Could you check a few things on this model? Use its own coordinates, in mm. Face numbers are marked on the shaded views. A direction names the side the tool comes from. Give positions to 0.01 mm unless a question says otherwise; leave off trailing zeros. Loops run counter-clockwise (first coordinate to the right, second up) from the corner with the lowest first, then second, coordinate; pieces in that order, holes last. Notation, with made-up numbers: (36.25, 40.25) - (58.25, 40.25) arc R10 ccw to (58.25, 57.25) - close; hole circle Ø5 at (74, -26.75). An arc over 180 degrees is marked (long way). One line per item, written item: value. Start each with the question number.
Q1. If I drill on line 1 (Z direction, x = 11, y = -428.5); line 2 (X direction, y = -446, z = 324.5); line 3 (Z direction, x = 118.5, y = -600), over which ranges is the centre line in solid material (lowest first)? Write a range as from..to.
Q2. I want a section at A-A (z = 465.5). Please give me the cut outline in (x, y), then the cut area to 3 significant figures.
Q3. I want a section at C-C (y = -469). Please give me the cut outline in (x, z), then the cut area to 3 significant figures.
Q4. For the marked faces 1, 2 and 3, which set-ups out of +Z, -Z, +X, -X, +Y, -Y let a thin tool reach every point of the face, with its end or its side?
Q5. I want a section at D-D (z = 618). Please give me the cut outline in (x, y).
Q6. I want a section at B-B (x = 69). Please give me the cut outline in (y, z), then the cut area to 3 significant figures.
Q7. I'm going to push flat-ended pins straight in: P1, Ø12, axis at x = -387.5, z = 736.5, coming from the -Y side; P2, Ø5, axis at x = 190, y = -269, coming from the -Z side. Where does each tip first touch, or does it pass through?
Q8. If we mould it in two halves opening along X, with no side actions, what happens to the marked faces 4, 5, 6 and 7? For each: released by +X, released by -X, zero draft, split by the parting line, or undercut.
```python
from build123d import *

# Parameters (mm, degrees)
F1_DEPTH  = 500
F3_W      = 50
F3_H      = 50
F4_DEPTH  = 650
F5_W      = 50
F5_H      = 50
F6_DEPTH  = 200
F8_W      = 1200
F8_H      = 18
F9_DEPTH  = 150
F11_DEPTH = 1164


with BuildPart() as f1:
    # F0 (on Front) → F1 (new body)
    with BuildSketch(Plane.XZ):
        Polygon((0, 1115), (-600, 1115), (-600, 200), (0, 200), (0, 218), (-582, 218), (-582, 1097), (0, 1097), align=None)
    extrude(amount=F1_DEPTH)

    # F3 (on offset) → F4 (join)
    with BuildSketch(Plane.XZ):
        with Locations((-575, 175)):
            Rectangle(F3_W, F3_H)
    extrude(amount=F4_DEPTH)

    # F5 (on Top) → F6 (join)
    with BuildSketch(Plane.XY):
        with Locations((-575, -25)):
            Rectangle(F5_W, F5_H)
        with Locations((-575, -625)):
            Rectangle(F5_W, F5_H)
    extrude(amount=F6_DEPTH)

    # F7: F1 across plane


with BuildPart() as f1_1:
    add(f1.part)
    add(f1.part.mirror(Plane.YZ))

    # F8 (on face) → F9 (join)
    with BuildSketch(Plane.XZ.offset(500)):
        with Locations((0, 1106)):
            Rectangle(F8_W, F8_H)
    extrude(amount=F9_DEPTH)

    # F10 (on face) → F11 (join, through all)
    with BuildSketch(Plane.YZ.offset(-582)):
        Polygon((0, 897), (-500, 897), (-500, 879), (-18, 879), (-18, 568), (-500, 568), (-500, 550), (0, 550), align=None)
    extrude(amount=F11_DEPTH)


solid = f1_1.part
```
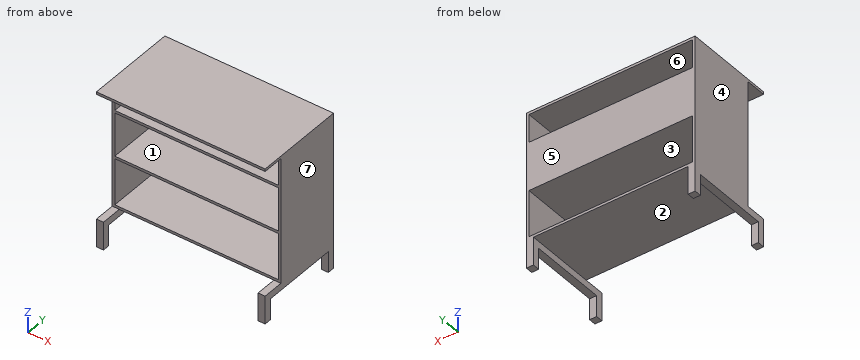
Worked answers:
1. line 1: z = 200..218, 550..568, 879..897, 1097..1115
1. line 2: x = -600..-582, 582..600
1. line 3: z = 1097..1115
2. outline: (-600, -500) - (-582, -500) - (-582, 0) - (-600, 0) - close; (582, -500) - (600, -500) - (600, 0) - (582, 0) - close
2. area: 18,000 mm²
3. outline: (-600, 150) - (-550, 150) - (-550, 200) - (550, 200) - (550, 150) - (600, 150) - (600, 1115) - (-600, 1115) - close; hole (-582, 218) - (582, 218) - (582, 550) - (-582, 550) - close; hole (-582, 568) - (582, 568) - (582, 879) - (-582, 879) - close; hole (-582, 897) - (582, 897) - (582, 1097) - (-582, 1097) - close
3. area: 122,000 mm²
4. face 1: -Y
4. face 2: -Z, +Y, -Y
4. face 3: +Y, -Y
5. outline: (-600, -500) - (-582, -500) - (-582, -18) - (582, -18) - (582, -500) - (600, -500) - (600, 0) - (-600, 0) - close
6. outline: (-650, 1097) - (0, 1097) - (0, 1115) - (-650, 1115) - close; (-500, 200) - (0, 200) - (0, 218) - (-500, 218) - close; (-500, 550) - (0, 550) - (0, 897) - (-500, 897) - (-500, 879) - (-18, 879) - (-18, 568) - (-500, 568) - close
6. area: 44,300 mm²
7. P1: stops at y = -18
7. P2: stops at z = 200
8. face 4: released by -X
8. face 5: zero draft
8. face 6: undercut
8. face 7: released by +X
